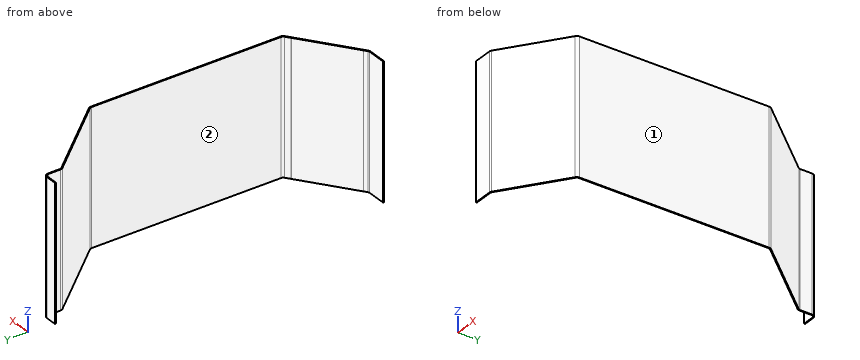
Autodesk Inventor part; units mm, degrees
ref_plane "YZ Plane" through (0, 0, 0) normal (1, 0, 0) x (0, 1, 0)
ref_plane "XZ Plane" through (0, 0, 0) normal (0, 1, 0) x (-1, 0, 0)
ref_plane "XY Plane" through (0, 0, 0) normal (0, 0, 1) x (1, 0, 0)
sketch "Sketch1" plane through (0, 0, 0) normal (0, 0, 1) x (1, 0, 0)
  line L0 (12.58, -266.7) -> (12.58, -12.7)
  line L1 (12.6094, 30.4615) -> (-104.0379, 164.6489)
  line L2 (-101.051, 167.6239) -> (-101.051, 171.0791)
  line L3 (-101.051, 183.7761) -> (-101.051, 187.2313)
  line L4 (2.2104, -312.663) -> (11.2162, -295.0088)
  line L5 (2.2104, -312.663) -> (-30.82, -336.6137)
  line L6 (-87.8643, -376.8499) -> (-98.4679, -380.082)
  line L7 (2.14, -312.5659) -> (-85.2529, -375.9353)
  line L8 (-103.9473, -380.8694) -> (-107.4025, -380.8694)
  line L9 (-120.0995, -380.8694) -> (-123.5547, -380.8694)
  line L10 (-120.0995, 190.1276) -> (-123.5547, 190.1276) construction
  line L11 (-101.051, 189.8019) -> (-116.705, 189.8019) construction
  line L12 (-126.451, -355.4694) -> (-126.451, 254.1306) construction
  line L13 (-126.451, 189.8019) -> (-101.051, 189.8019)
  line L14 (12.6094, 30.4615) -> (12.6094, -304.9744)
  line L15 (12.6094, -304.9744) -> (-92.0576, -380.8694)
  line L16 (-92.0576, -380.8694) -> (-126.451, -380.8694)
  line L17 (12.6094, 30.4615) -> (-101.051, 161.2129)
  line L18 (-101.051, 161.2129) -> (-101.051, 189.8019)
  line L19 (-126.451, 191.4275) -> (-99.4254, 191.4275)
  line L20 (-99.4254, 191.4275) -> (-99.4254, 161.8207)
  line L21 (-99.4254, 161.8207) -> (14.235, 31.0693)
  line L22 (14.235, 31.0693) -> (14.235, -305.8037)
  line L23 (14.235, -305.8037) -> (-91.5302, -382.495)
  line L24 (-91.5302, -382.495) -> (-126.451, -382.495)
  line L25 (-126.451, 189.8019) -> (-126.451, 191.4275)
  line L26 (-126.451, -382.495) -> (-126.451, -380.8694)
  point P0 (0, 0)
  dimension "d0" = 1.6256
extrude "Extrusion1" add sketch "Sketch1" against normal blind 234
fillet "Fillet1" radius 5 5 edges at (-101.051, 189.8019, -117) (-99.4254, 161.8207, -117) (12.6094, 30.4615, -117) (12.6094, -304.9744, -117) (-92.0576, -380.8694, -117)
fillet "Fillet2" radius 7 5 edges at (-91.5302, -382.495, -117) (14.235, -305.8037, -117) (14.235, 31.0693, -117) (-101.051, 161.2129, -117) (-99.4254, 191.4275, -117)
properties part number "skidPlateV1" material "Stainless Steel"
Could you check a few things on this model? Use its own coordinates, in mm. Face numbers are marked on the shaded views. A direction names the side the tool comes from. Give positions to 0.01 mm unless a question says otherwise; leave off trailing zeros. Order: outer loops, then holes, each group sorted by start corner. A loop starts at its lowest first (then second) coordinate and runs counter-clockwise, first axis right, second up.
Q1. Suppose I cut it at A-A, the plane x = -19.5. Write out the boundary of the cut face in (y, z).
Q2. Suppose I cut it at B-B, the plane y = -34.5. Write out the boundary of the cut face in (x, z) (3 decimals).
Q3. I'm going to push flat-ended pins straight in: P1, Ø4, axis at x = -47.5, z = -172.5, coming from the -Y side; P2, Ø3, axis at y = 30, z = -173.5, coming from the -X side; P3, Ø1.5, axis at y = 122.5, z = -70.5, coming from the +X side. Where does each tip first touch, or does it pass through?
Q4. For the marked faces 1 and 2, which set-ups out of +Z, -Z, +X, -X, +Y, -Y let a thin tool reach every point of the face, with its end or its side?
Q5. Suppose I cut it at C-C, the plane x = -77.5. Write out the boundary of the cut face in (y, z), and give its area (3 significant figures).
Q6. If I drill on line 1 along X through (y, z) = (-214.5, -180) (3 decimals); line 2 along Y through (x, z) = (-75, -191); line 3 along Y through (x, z) = (-9, -98.5), over which ranges is the centre line in solid material (lowest first)?
Q7. Suppose I cut it at D-D, the plane y = 134.5. Write out the boundary of the cut face in (x, z), and give its area (3 significant figures).
Solution:
1. outline: (-330.27, -234) - (-328.26, -234) - (-328.26, 0) - (-330.27, 0) - close; (67.4, -234) - (69.88, -234) - (69.88, 0) - (67.4, 0) - close
2. outline: (12.609, -234) - (14.235, -234) - (14.235, 0) - (12.609, 0) - close
3. P1: stops at y = -352.02
3. P2: stops at x = 11.68
3. P3: stops at x = -64.59
4. face 1: +Z, -Z, +X, +Y, -Y
4. face 2: +Z, -Z, -X
5. outline: (-372.32, -234) - (-370.31, -234) - (-370.31, 0) - (-372.32, 0) - close; (134.12, -234) - (136.6, -234) - (136.6, 0) - (134.12, 0) - close
5. area: 1,050 mm2
6. line 1: x = 12.609 to 14.235
6. line 2: y = -370.51 to -368.5, 131.24 to 133.72
6. line 3: y = -322.65 to -320.64, 55.32 to 57.8
7. outline: (-77.83, -234) - (-75.68, -234) - (-75.68, 0) - (-77.83, 0) - close
7. area: 504 mm2
